CAD build for the part. Positions are in the model's coordinates, mm. A direction names the side the tool comes from. Give positions to 0.01 mm unless a question says otherwise; leave off trailing zeros. Loops run counter-clockwise (first coordinate to the right, second up) from the corner with the lowest first, then second, coordinate; pieces in that order, holes last.
Item 1: Saw through at B-B on y = 12.25. Give the cut face in (x, z), plus the area to 3 significant figures.
Item 2: Probe probe 1 along Y at (x, z) = (8.75, 2.1); probe 2 along X at (y, z) = (-0.25, 2.8); probe 3 along Y at (x, z) = (4.75, 1.3). List the from-to ranges inside material, lowest first.
Item 3: Saw through at A-A on z = 1. Give the cut face in (x, y).
Item 4: Saw through at C-C on x = 1. Give the cut face in (y, z).
Item 5: Mould opens along Y. For faces 1 (the flat face through (0, -1, 1)), 2 (the flat face through (9, 14, 2)), 3 (the flat face through (6, 0, 1)) say: released by +Y, released by -Y, zero draft, split by the parting line, or undercut.
Item 6: Which spindle directions (+Z, -Z, +X, -X, +Y, -Y) get a long thin tool onto all of the face, cutting with end or side? Do faces 4 (the flat face through (5, 5, 3)), 5 (the flat face through (4, -1, 1)). Say none if no direction does.
Item 7: Drop flat-ended pins along their axis: P1, Ø0.9, axis at x = 5, z = 2, coming from the -Y side; P2, Ø1.5, axis at x = 4, y = 12, coming from the -Z side; P3, Ø0.9, axis at y = 5, z = 1, coming from the +X side; P4, Ø1.5, axis at x = 9, z = 1.5, coming from the -Y side. Give the stop position or say it passes through.
from build123d import *

# Parameters (mm, degrees)
EXTRUDE_1_DEPTH = 3
SKETCH_2_W      = 4
SKETCH_2_H      = 3
EXTRUDE_2_DEPTH = 3
SKETCH_3_W      = 3
SKETCH_3_H      = 7
EXTRUDE_3_DEPTH = 3


with BuildPart() as part:
    # 草图1 → 凸台-拉伸1 (new body)
    with BuildSketch(Plane.XY):
        Polygon((0, 0), (8, 0), (8, 14), align=None)
    extrude(amount=EXTRUDE_1_DEPTH)

    # 草图2 → 凸台-拉伸2 (add)
    with BuildSketch(Plane.XZ):
        with Locations((2, 1.5)):
            Rectangle(SKETCH_2_W, SKETCH_2_H)
    extrude(amount=EXTRUDE_2_DEPTH)

    # 草图3 → 凸台-拉伸3 (add)
    with BuildSketch(Plane(origin=(8, 0, 0), x_dir=(0, 0, -1), z_dir=(1, 0, 0))):
        with Locations((-1.5, 10.5)):
            Rectangle(SKETCH_3_W, SKETCH_3_H)
    extrude(amount=EXTRUDE_3_DEPTH)


solid = part.part
Results below:
1. outline: (7, 0) - (11, 0) - (11, 3) - (7, 3) - close
1. area: 12.0 mm2
2. probe 1: y = 7 to 14
2. probe 2: x = 0 to 4
2. probe 3: y = 0 to 8.31
3. outline: (0, -3) - (4, -3) - (4, 0) - (8, 0) - (8, 7) - (11, 7) - (11, 14) - (8, 14) - (0, 0) - close
4. outline: (-3, 0) - (1.75, 0) - (1.75, 3) - (-3, 3) - close
5. face 1: zero draft
5. face 2: released by +Y
5. face 3: released by -Y
6. face 4: +Z, +X, -X, +Y, -Y
6. face 5: +Z, -Z, +X, -Y
7. P1: stops at y = 0
7. P2: passes through
7. P3: stops at x = 8
7. P4: stops at y = 7
